Source: CAD feature listing. Evaluate the final solid. Frame: model axes, mm. Coordinates: 2 decimals unless noted, no trailing zeros. Order: outer loops, then holes, each group sorted by start corner. A loop starts at its lowest first (then second) coordinate and runs counter-clockwise, first axis right, second up.
```python
from build123d import *

# Parameters (mm, degrees)
F0_W     = 127
F0_H     = 95
F1_DEPTH = 5
F2_R     = 2.1
F3_DEPTH = 5.001
F4_R     = 4.99999


# Not quite as in the source:
# - a fillet or chamfer is up to 0.001 mm smaller than in the source, because OpenCascade refuses the exact size


with BuildPart() as f1:
    # F0 (on Top) → F1 (new body)
    with BuildSketch(Plane.XY):
        with Locations((1.5311012896, -0.0675843805)):
            Rectangle(F0_W, F0_H)
    extrude(amount=F1_DEPTH)

    # F2 (on face) → F3 (cut, through all)
    with BuildSketch(Plane.XY.offset(5)):
        with Locations((-46.9688987104, 32.4324156195)):
            Circle(F2_R)
        with Locations((-46.9688987104, -32.5675843805)):
            Circle(F2_R)
        with Locations((50.0311012896, -32.5675843805)):
            Circle(F2_R)
    extrude(amount=-F3_DEPTH, mode=Mode.SUBTRACT)

    # F4 (radius 5 in the source; OpenCascade refuses exactly that, so slightly less here)
    f4_edges = [f1.edges().sort_by_distance(p)[0] for p in [
        (1.531101, 47.432416, 5),
        (65.031101, -0.067584, 5),
        (-61.968899, -0.067584, 5),
        (1.531101, -47.567584, 5),
        (-61.968899, -47.567584, 2.5),
        (-61.968899, 47.432416, 2.5),
        (65.031101, 47.432416, 2.5),
        (65.031101, -47.567584, 2.5),
    ]]
    fillet(f4_edges, radius=F4_R)


solid = f1.part
```
1. Draft query along X for faces 1 (the face through (1, 1, 5)), 2 (the face through (-44.966, -31.937, 2.535)), 3 (the face through (63.5, 0.5, 3.6)). Return one class per face: released by +X, released by -X, zero draft, split by the parting line, or undercut.
Findings:
face 1: zero draft
face 2: undercut
face 3: released by +X
2. Section query B-B on z = 2.4. Return loops of the section in (x, y).
Findings:
outline: (-61.36, -42.57) arc R4.39 ccw to (-56.97, -46.95) - (60.03, -46.95) arc R4.39 ccw to (64.42, -42.57) - (64.42, 42.43) arc R4.39 ccw to (60.03, 46.82) - (-56.97, 46.82) arc R4.39 ccw to (-61.36, 42.43) - close; hole circle Ø4.2 at (-46.97, -32.57); hole circle Ø4.2 at (-46.97, 32.43); hole circle Ø4.2 at (50.03, -32.57)
3. Ray query, line 1 (Y direction, x = 30.5, z = 2) (3 decimals); line 2 (X direction, y = 42, z = 0.65); line 3 (X direction, y = -0.5, z = 4.5). Return the intervals inside material, ascending.
Findings:
line 1: y = -47.15 to 47.015
line 2: x = -61.93 to 64.99
line 3: x = -59.15 to 62.21
4. Pin query (flat end, axial travel): P1, Ø2, axis at x = -36.5, z = 1.5, coming from the +Y side; P2, Ø5.5, axis at x = -46.97, y = 32.43, coming from the +Z side; P3, Ø1, axis at y = 22, z = 1, coming from the +X side. Return the tip coordinate at first contact, or that it passes through.
Findings:
P1: stops at y = 47.41
P2: stops at z = 5
P3: stops at x = 65.01
